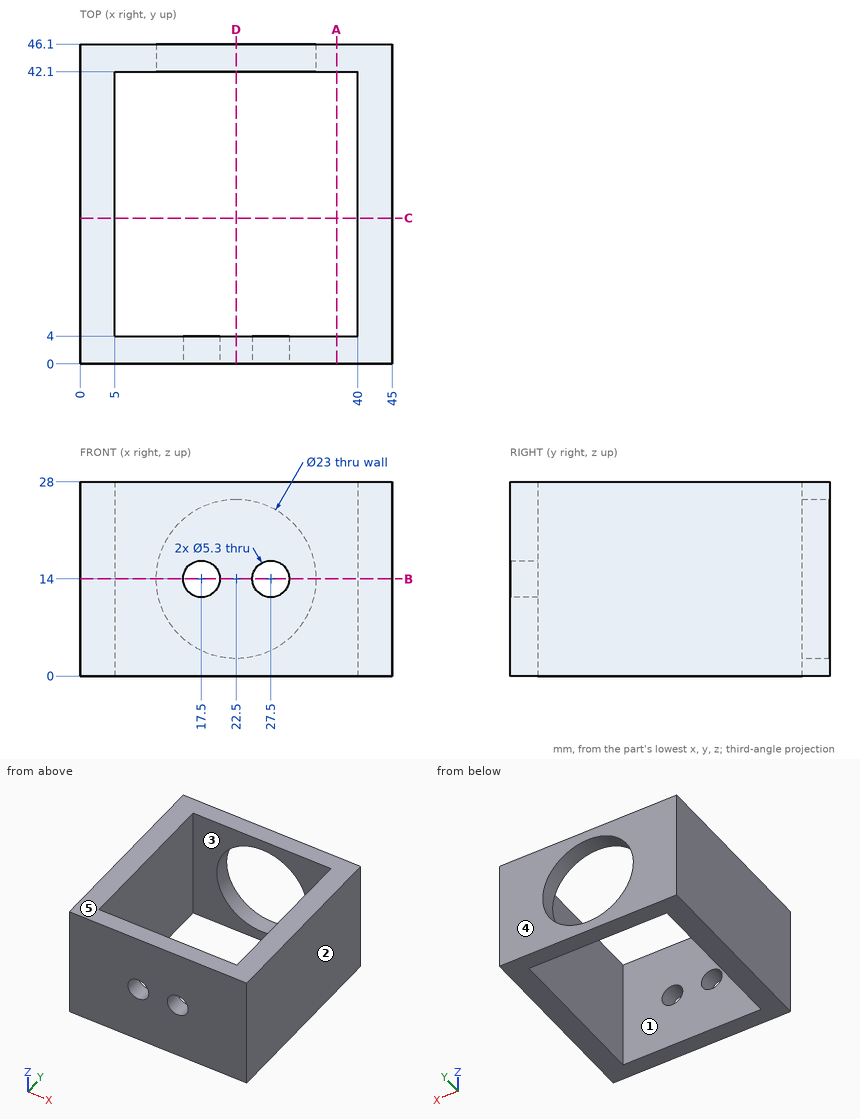
Drawing for the job (mm, zero at the part's lowest x, y, z). A direction names the side the tool comes from. Coordinates: 2 decimals unless noted, no trailing zeros. Loops run counter-clockwise (first coordinate to the right, second up) from the corner with the lowest first, then second, coordinate; pieces in that order, holes last. Notation, with made-up numbers: (20.5, 18.25) - (54.5, 18.25) arc R19 cw to (54.5, 29.25) - close; hole circle Ø2 at (20, 30.5). An arc over 180 degrees is marked (long way). Return JSON: item names as keys, results as strings.
1. Band-saw the part on D-D (x = 22.5). Give the cut face in (y, z).
Result:
{"outline": "(0, 0) - (4, 0) - (4, 28) - (0, 28) - close; (42.1, 0) - (46.1, 0) - (46.1, 2.5) - (42.1, 2.5) - close; (42.1, 25.5) - (46.1, 25.5) - (46.1, 28) - (42.1, 28) - close"}
2. Mould opens along Y. For the marked faces 3, 4 and 5 say: released by +Y, released by -Y, zero draft, split by the parting line, or undercut.
Result:
{"face 3": "undercut", "face 4": "released by +Y", "face 5": "zero draft"}
3. Band-saw the part on A-A (x = 37). Give the cut face in (y, z).
Result:
{"outline": "(0, 0) - (4, 0) - (4, 28) - (0, 28) - close; (42.1, 0) - (46.1, 0) - (46.1, 28) - (42.1, 28) - close"}
4. Drop a flat-ended pin along its axis: pin 1 (4 mm diameter, centred on x = 15, z = 17.5, fed in from +Y). Give the stop position or say it passes through.
Result:
{"pin 1": "stops at y = 4"}
5. Probe L1, parallel to X at y = 3.25, z = 14; L2, parallel to X at y = 43.7, z = 14; L3, parallel to X at y = 22.5, z = 10.75. List the from-to ranges inside material, lowest first. Write a range as from..to.
Result:
{"L1": "x = 0..14.85, 20.15..24.85, 30.15..45", "L2": "x = 0..11, 34..45", "L3": "x = 0..5, 40..45"}
6. 3-axis set-ups, long thin cutter, end or side, ignore diameter. For the marked faces 1 and 2: which of +Z, -Z, +X, -X, +Y, -Y reach the whole face in a straight line?
Result:
{"face 1": "+Z, -Z", "face 2": "+Z, -Z, +X, +Y, -Y"}
7. Band-saw the part on C-C (y = 21). Give the cut face in (x, z), and give its area (3 significant figures).
Result:
{"outline": "(0, 0) - (5, 0) - (5, 28) - (0, 28) - close; (40, 0) - (45, 0) - (45, 28) - (40, 28) - close", "area": "280 mm2"}
8. Band-saw the part on B-B (z = 14). Give the cut face in (x, y).
Result:
{"outline": "(0, 0) - (14.85, 0) - (14.85, 4) - (5, 4) - (5, 42.1) - (11, 42.1) - (11, 46.1) - (0, 46.1) - close; (20.15, 0) - (24.85, 0) - (24.85, 4) - (20.15, 4) - close; (30.15, 0) - (45, 0) - (45, 46.1) - (34, 46.1) - (34, 42.1) - (40, 42.1) - (40, 4) - (30.15, 4) - close"}
